from build123d import *

# Parameters (mm, degrees)
F0_R     = 10
F1_DEPTH = 5
F3_DEPTH = 5
F4_R     = 7.5
F5_DEPTH = 5
F7_DEPTH = 5
F8_R     = 1.25
F9_DEPTH = 5


with BuildPart() as f1:
    # F0 (on Top) → F1 (new body)
    with BuildSketch(Plane.XY):
        Circle(F0_R)
    extrude(amount=F1_DEPTH)

    # F2 (on Top) → F3 (join)
    with BuildSketch(Plane.XY):
        Polygon((-2.5, 25), (-8.5, 0), (8.5, 0), (2.5, 25), align=None)
    extrude(amount=F3_DEPTH)

    # F4 (on Top) → F5 (cut)
    with BuildSketch(Plane.XY):
        Circle(F4_R)
    extrude(amount=F5_DEPTH, mode=Mode.SUBTRACT)

    # F6 (on Top) → F7 (cut)
    with BuildSketch(Plane.XY):
        Polygon((19.809051, -7.209905), (0, 0), (-19.809051, -7.209905), (0, -14.41981), align=None)
    extrude(amount=F7_DEPTH, mode=Mode.SUBTRACT)

    # F8 (on Top) → F9 (cut)
    with BuildSketch(Plane.XY):
        with Locations((0, 20)):
            Circle(F8_R)
    extrude(amount=F9_DEPTH, mode=Mode.SUBTRACT)


solid = f1.part
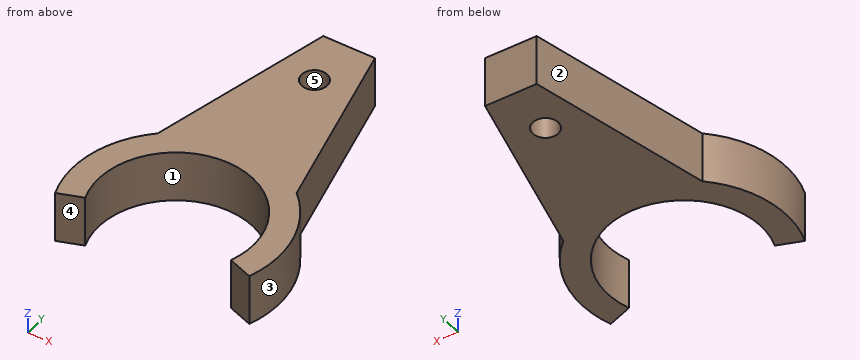
For this review, take the finished solid that the model builds, in its own axes (mm). Face numbers are marked on the shaded views. A direction names the side the tool comes from. Round coordinates to 2 decimals unless told otherwise and drop trailing zeros. Loops run counter-clockwise (first coordinate to the right, second up) from the corner with the lowest first, then second, coordinate; pieces in that order, holes last. Notation, with made-up numbers: (65, -32) - (116, -32) arc R9 cw to (116, -22) - close; hole circle Ø3 at (20.5, -11). An arc over 180 degrees is marked (long way). Use one line per item in the form item = value.
1) Mouldability with a two-part tool opening along X and no side actions: class the marked faces 1, 2 and 3 as pulls with the +X half, pulls with the -X half, needs draft (parallel to the pull), parting line crosses it, or undercut.
Solutions:
face_1 = undercut
face_2 = pulls with the -X half
face_3 = pulls with the +X half
2) Clearance check with flat-ended pins moving along their axes: P1, Ø4, axis at x = -5.5, y = 20.5, coming from the -Z side; P2, Ø1.5, axis at y = 7, z = 2, coming from the -X side; P3, Ø2, axis at x = -2, z = 2, coming from the -Y side. State where each tip first meets the part, or that it passes through.
Solutions:
P1 = 0
P2 = -7.81
P3 = 6.87
3) We need section C-C on z = 0.9. Write out the cut boundary in (x, y).
Solutions:
outline = (-9.4, -3.42) - (-7.05, -2.57) arc R7.5 cw (long way) to (7.05, -2.57) - (9.4, -3.42) arc R10 ccw to (6.72, 7.4) - (2.5, 25) - (-2.5, 25) - (-6.72, 7.4) arc R10 ccw to start; hole circle Ø2.5 at (0, 20)
4) We need section D-D on y = 23. Write out the cut boundary in (x, z), then the cut area to 3 significant figures.
Solutions:
outline = (-2.98, 0) - (2.98, 0) - (2.98, 5) - (-2.98, 5) - close
area = 29.8 mm2
5) We need section B-B on y = 20. Write out the cut boundary in (x, z).
Solutions:
outline = (-3.7, 0) - (-1.25, 0) - (-1.25, 5) - (-3.7, 5) - close; (1.25, 0) - (3.7, 0) - (3.7, 5) - (1.25, 5) - close
6) We need section A-A on x = 0. Write out the cut boundary in (y, z), then the cut area to 3 significant figures.
Solutions:
outline = (7.5, 0) - (18.75, 0) - (18.75, 5) - (7.5, 5) - close; (21.25, 0) - (25, 0) - (25, 5) - (21.25, 5) - close
area = 75.0 mm2
7) Wall thickness on probe 1 along Y at (x, z) = (0, 2.95); probe 2 along X at (y, z) = (0, 3.1); probe 3 along X at (y, z) = (19.5, 3.3): over which ranges is each line inside the solid? List them lowest first.
Solutions:
probe_1 = 7.5 to 18.75, 21.25 to 25
probe_2 = -10 to -7.5, 7.5 to 10
probe_3 = -3.82 to -1.15, 1.15 to 3.82
8) Tool access review of the marked faces 4 and 5: name each direction out of +Z, -Z, +X, -X, +Y, -Y from which nothing blocks a thin tool from reaching the whole face with its end or side.
Solutions:
face_4 = +Z, -Z, -Y
face_5 = +Z, -Z
